```python
from build123d import *

# Parameters (mm, degrees)
SKETCH1_W           = 30
SKETCH1_H           = 26.5
BOSS_EXTRUDE1_DEPTH = 2.5
SKETCH2_W           = 22
SKETCH2_H           = 2
BOSS_EXTRUDE2_DEPTH = 0.5
SKETCH3_W           = 26
SKETCH3_H           = 2
BOSS_EXTRUDE3_DEPTH = 1.5
SKETCH4_R           = 2
BOSS_EXTRUDE4_DEPTH = 2.5


with BuildPart() as part:
    # Sketch1 → Boss-Extrude1 (new, symmetric)
    with BuildSketch(Plane(origin=(-179.150792305, 0, 0), x_dir=(0, 0, -1), z_dir=(1, 0, 0))):
        with Locations((-149, 50.25)):
            Rectangle(SKETCH1_W, SKETCH1_H)
    extrude(amount=BOSS_EXTRUDE1_DEPTH, both=True)

    # Sketch2 → Boss-Extrude2 (add, symmetric)
    with BuildSketch(Plane(origin=(-181.650792305, 0, 0), x_dir=(0, 0, -1), z_dir=(1, 0, 0))):
        with Locations((-149, 41)):
            Rectangle(SKETCH2_W, SKETCH2_H)
        with Locations((-149, 45)):
            Rectangle(SKETCH2_W, SKETCH2_H)
    extrude(amount=BOSS_EXTRUDE2_DEPTH, both=True)

    # Sketch3 → Boss-Extrude3 (add, symmetric)
    with BuildSketch(Plane(origin=(-175.150792305, 0, 0), x_dir=(0, 0, -1), z_dir=(1, 0, 0))):
        with Locations((-149, 62.5)):
            Rectangle(SKETCH3_W, SKETCH3_H)
    extrude(amount=BOSS_EXTRUDE3_DEPTH, both=True)

    # Sketch4 → Boss-Extrude4 (add, symmetric)
    with BuildSketch(Plane(origin=(-174.150792305, 0, 0), x_dir=(0, 0, -1), z_dir=(1, 0, 0))):
        with Locations((-149, 43)):
            Circle(SKETCH4_R)
    extrude(amount=BOSS_EXTRUDE4_DEPTH, both=True)


solid = part.part
```
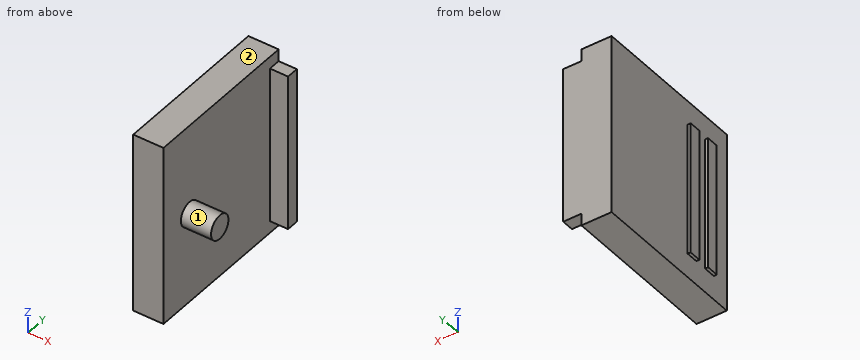
Model file for the job. Use its own axes, mm. Face numbers are marked on the shaded views. A direction names the side the tool comes from. Round coordinates to 2 decimals unless told otherwise and drop trailing zeros. Write each loop counter-clockwise with the first axis right and the second up, starting at its lowest first coordinate (ties: lowest second). Pieces come first, ordered by that corner, then holes. Notation, with made-up numbers: M -27.5,-18.75 L -8.5,-18.75 A30 ccw -8.5,5.25 Z; hole C 3.5,80.5 d1. An arc over 180 degrees is marked long. Put each result on its own line as item: value.
Item 1: Flat gauge pins, fed straight in: P1, Ø0.6, axis at x = -182, z = 146.5, coming from the -Y side; P2, Ø2, axis at y = 62.5, z = 155.5, coming from the +X side; P3, Ø2, axis at y = 47.5, z = 154.5, coming from the +X side. Where does each tip first touch, or does it go through?
Responses:
P1: y = 40
P2: x = -173.65
P3: x = -176.65
Item 2: Cut at B-B (x = -175.75). List the corners of the cut face in (y, z), and give its area (3 significant figures).
Responses:
outline: C 43,149 d4; M 61.5,136 L 63.5,136 L 63.5,162 L 61.5,162 Z
area: 64.6 mm²
Item 3: Cut at D-D (x = -173). List the corners of the cut face in (y, z), and give its area (3 significant figures).
Responses:
outline: C 43,149 d4
area: 12.6 mm²
Item 4: Tool access for the marked faces 1 and 2: list every direction of +Z, -Z, +X, -X, +Y, -Y with a clear straight run to the whole face (end or side of a thin tool).
Responses:
face 1: +X
face 2: +Z, +X, -X, +Y, -Y
Item 5: Cut at A-A (y = 40.5). List the corners of the cut face in (x, z), and give its area (3 significant figures).
Responses:
outline: M -182.15,138 L -181.65,138 L -181.65,134 L -176.65,134 L -176.65,164 L -181.65,164 L -181.65,160 L -182.15,160 Z
area: 161 mm²
Item 6: Probe L1, parallel to X at y = 39.25, z = 154; L2, parallel to X at y = 62, z = 142; L3, parallel to Y at x = -174, z = 150. List the from-to ranges inside material, lowest first. Write a range as from..to.
Responses:
L1: -181.65..-176.65
L2: -181.65..-173.65
L3: 41.27..44.73, 61.5..63.5
Item 7: Cut at C-C (z = 146.5). List the corners of the cut face in (x, y).
Responses:
outline: M -182.15,40 L -181.65,40 L -181.65,37 L -176.65,37 L -176.65,61.5 L -173.65,61.5 L -173.65,63.5 L -181.65,63.5 L -181.65,46 L -182.15,46 L -182.15,44 L -181.65,44 L -181.65,42 L -182.15,42 Z
